Can you work these out from the model? Positions are in its coordinate system, mm. A direction names the side the tool comes from. Round coordinates to 2 decimals unless told otherwise and drop trailing zeros. Order: outer loops, then holes, each group sorted by start corner. A loop starts at its lowest first (then second) coordinate and runs counter-clockwise, first axis right, second up. Notation, with made-up numbers: (60, 19) -> (107, 19) arc R23 ccw to (107, 42) -> close; hole circle Ø3 at (-24, -32). An arc over 180 degrees is marked (long way). One line per item, written item: value.
```python
from build123d import *

# Parameters (mm, degrees)
SKETCH1_W          = 25.4
SKETCH1_H          = 76.2
EXTRUDE1_DEPTH     = 3.175
SKETCH3_W          = 3.175
SKETCH3_H          = 6.35
CUT_EXTRUDE1_DEPTH = 3.175
LPATTERN1_COUNT    = 3
LPATTERN1_PITCH    = 69.85
SKETCH4_W          = 3.175
SKETCH4_H          = 12.7
CUT_EXTRUDE2_DEPTH = 3.175
LPATTERN2_COUNT    = 2
LPATTERN2_PITCH    = 25.4
SKETCH5_W          = 12.7
SKETCH5_H          = 3.175
CUT_EXTRUDE3_DEPTH = 3.175
SKETCH6_W          = 6.35
SKETCH6_H          = 3.175
CUT_EXTRUDE4_DEPTH = 3.175
LPATTERN3_COUNT    = 2
LPATTERN3_PITCH    = 19.05


with BuildPart() as part:
    # Sketch1 → Extrude1 (new body)
    with BuildSketch(Plane.XY):
        with Locations((12.7, 38.1)):
            Rectangle(SKETCH1_W, SKETCH1_H)
    extrude(amount=EXTRUDE1_DEPTH)

    # Sketch3 → Cut-Extrude1 (cut)
    with BuildSketch(Plane.XY.offset(3.175)):
        with Locations((23.8125, 73.025)):
            Rectangle(SKETCH3_W, SKETCH3_H)
    cut_extrude1 = extrude(amount=-CUT_EXTRUDE1_DEPTH, mode=Mode.SUBTRACT)

    # LPattern1: Cut-Extrude1 ×3
    with Locations(*[(0, -i * LPATTERN1_PITCH, 0) for i in range(1, LPATTERN1_COUNT)]):
        add(cut_extrude1, mode=Mode.SUBTRACT)

    # Sketch4 → Cut-Extrude2 (cut)
    with BuildSketch(Plane.XY.offset(3.175)):
        with Locations((23.8125, 50.8)):
            Rectangle(SKETCH4_W, SKETCH4_H)
    cut_extrude2 = extrude(amount=-CUT_EXTRUDE2_DEPTH, mode=Mode.SUBTRACT)

    # LPattern2: Cut-Extrude2 ×2
    with Locations(*[(0, -i * LPATTERN2_PITCH, 0) for i in range(1, LPATTERN2_COUNT)]):
        add(cut_extrude2, mode=Mode.SUBTRACT)

    # Sketch5 → Cut-Extrude3 (cut)
    with BuildSketch(Plane.XY.offset(3.175)):
        with Locations((12.7, 1.5875)):
            Rectangle(SKETCH5_W, SKETCH5_H)
    extrude(amount=-CUT_EXTRUDE3_DEPTH, mode=Mode.SUBTRACT)

    # Sketch6 → Cut-Extrude4 (cut)
    with BuildSketch(Plane.XY.offset(3.175)):
        with Locations((3.175, 74.6125)):
            Rectangle(SKETCH6_W, SKETCH6_H)
    cut_extrude4 = extrude(amount=-CUT_EXTRUDE4_DEPTH, mode=Mode.SUBTRACT)

    # LPattern3: Cut-Extrude4 ×2
    with Locations(*[(i * LPATTERN3_PITCH, 0, 0) for i in range(1, LPATTERN3_COUNT)]):
        add(cut_extrude4, mode=Mode.SUBTRACT)


solid = part.part
```
Q1. I want a section at A-A on z = 0.95. List the corners of the cut face in (x, y) for me (3 decimals).
Answers below:
outline: (0, 0) -> (6.35, 0) -> (6.35, 3.175) -> (19.05, 3.175) -> (19.05, 0) -> (22.225, 0) -> (22.225, 6.35) -> (25.4, 6.35) -> (25.4, 19.05) -> (22.225, 19.05) -> (22.225, 31.75) -> (25.4, 31.75) -> (25.4, 44.45) -> (22.225, 44.45) -> (22.225, 57.15) -> (25.4, 57.15) -> (25.4, 69.85) -> (22.225, 69.85) -> (22.225, 73.025) -> (19.05, 73.025) -> (19.05, 76.2) -> (6.35, 76.2) -> (6.35, 73.025) -> (0, 73.025) -> close
Q2. I want a section at C-C on y = 50.5. List the corners of the cut face in (x, z) for me (3 decimals).
Answers below:
outline: (0, 0) -> (22.225, 0) -> (22.225, 3.175) -> (0, 3.175) -> close
Q3. Will these pins go through, and if not, where does the flat tip stop? pin 1 Ø1.6 at (x, z) = (2.5, 2) entering from +Y (3 decimals); pin 2 Ø1 at (x, z) = (24, 2) entering from +Y; pin 3 Ø1.6 at (y, z) = (71, 1.5) entering from +X (3 decimals).
Answers below:
pin 1: y = 73.025
pin 2: y = 69.85
pin 3: x = 22.225
Q4. On a 3-axis mill with a long thin cutter (end or side, diameter ignored), from which of +Z, -Z, +X, -X, +Y, -Y can I reach the whole of each face in a straight line? I mean faces 4 (the face through (22.225, 71, 2)), 5 (the face through (13, 3.175, 2)), 6 (the face through (24, 6.35, 2)), 7 (the face through (24, 44.45, 2)), 8 (the face through (6.35, 75, 2)). Say none if no direction works.
Answers below:
face 4: +Z, -Z, +X, +Y
face 5: +Z, -Z, -Y
face 6: +Z, -Z, +X, -Y
face 7: +Z, -Z, +X
face 8: +Z, -Z, -X, +Y
Q5. I want a section at B-B on x = 20. List the corners of the cut face in (y, z) for me (3 decimals), plus the area to 3 significant figures.
Answers below:
outline: (0, 0) -> (73.025, 0) -> (73.025, 3.175) -> (0, 3.175) -> close
area: 232 mm^2
Q6. We'd pull the mould along Y, two halves only. Please class faces 1 (the face through (24, 69.85, 2)), 2 (the face through (13, 39, 3.175)), 3 (the face through (22.225, 25, 2)): released by +Y, released by -Y, zero draft, split by the parting line, or undercut.
Answers below:
face 1: released by +Y
face 2: zero draft
face 3: undercut
Q7. Please list where these lines run through material, in increasing order: line 1 along Y through (x, z) = (9.5, 0.25) (3 decimals); line 2 along X through (y, z) = (30, 1.55) (3 decimals); line 3 along Y through (x, z) = (6, 0.65) (3 decimals).
Answers below:
line 1: 3.175 to 76.2
line 2: 0 to 22.225
line 3: 0 to 73.025
